Build history of the part. All positions in model axes, mm. A direction names the side the tool comes from. Give positions to 0.01 mm unless a question says otherwise; leave off trailing zeros. Write each loop counter-clockwise with the first axis right and the second up, starting at its lowest first coordinate (ties: lowest second). Pieces come first, ordered by that corner, then holes.
from build123d import *

# Parameters (mm, degrees)
SKETCH_1_R          = 20
SKETCH_1_R_2        = 5
SKETCH_1_R_3        = 2.25
EXTRUDE_1_DEPTH     = 6
SKETCH_2_R          = 9.5
SKETCH_2_R_2        = 5
EXTRUDE_2_DEPTH     = 23
SKETCH_3_R          = 3.75
CUT_EXTRUDE_1_DEPTH = 4.5


with BuildPart() as part:
    # Эскиз1 → Бобышка-Вытянуть1 (new body)
    with BuildSketch(Plane.XY):
        Circle(SKETCH_1_R)
        Circle(SKETCH_1_R_2, mode=Mode.SUBTRACT)
        with Locations((0, 14.5)):
            Circle(SKETCH_1_R_3, mode=Mode.SUBTRACT)
        with Locations((14.5, 0)):
            Circle(SKETCH_1_R_3, mode=Mode.SUBTRACT)
        with Locations((0, -14.5)):
            Circle(SKETCH_1_R_3, mode=Mode.SUBTRACT)
        with Locations((-14.5, 0)):
            Circle(SKETCH_1_R_3, mode=Mode.SUBTRACT)
    extrude(amount=EXTRUDE_1_DEPTH)

    # Эскиз2 → Бобышка-Вытянуть2 (add)
    with BuildSketch(Plane.XY.offset(6)):
        Circle(SKETCH_2_R)
        Circle(SKETCH_2_R_2, mode=Mode.SUBTRACT)
    extrude(amount=EXTRUDE_2_DEPTH)

    # Эскиз3 → Вырез-Вытянуть1 (cut)
    with BuildSketch(Plane(origin=(0, 0, 0), x_dir=(-1, 0, 0), z_dir=(0, 0, -1))):
        with Locations((0, 14.5)):
            Circle(SKETCH_3_R)
        with Locations((14.5, 0)):
            Circle(SKETCH_3_R)
        with Locations((0, -14.5)):
            Circle(SKETCH_3_R)
        with Locations((-14.5, 0)):
            Circle(SKETCH_3_R)
    extrude(amount=-CUT_EXTRUDE_1_DEPTH, mode=Mode.SUBTRACT)


solid = part.part
(1) Saw through at A-A, the plane x = 0. List the corners of the cut face in (y, z).
(2) Mould opens along X. For faces 4 (the face through (4, -9, 6)), 5 (the face through (13, -2, 4.5)), 6 (the face through (-4.336, -19.524, 2.958)) say: +X half, -X half, draft (parallel to the pull), parting line (faces both ways), or undercut.
(3) Probe line 1 (Y direction, x = 0, z = 2); line 2 (Y direction, x = 0, z = 4.9); line 3 (Z direction, x = -8.5, y = 12.5). List the from-to ranges inside material, lowest first.
(4) Drop flat-ended pins along their axis: pin 1 (8.5 mm diameter, centred on x = 14.5, y = 0, fed in from +Z); pin 2 (6 mm diameter, centred on x = -14.5, z = 6, fed in from -Y); pin 3 (5 mm diameter, centred on y = 11, z = 14, fed in from +X); pin 4 (3.5 mm diameter, centred on x = 0, y = -14.5, fed in from +Z). Give the stop position or say it passes through.
(5) Saw through at B-B, the plane y = 14.5. List the corners of the cut face in (x, z), plus the area to 3 significant figures.
(6) 3-axis set-ups, long thin cutter, end or side, ignore diameter. For faces 1 (the face through (-0.488, -16.696, 5.24)), 2 (the face through (4.38, -8.43, 17.34)), 3 (the face through (-2, -16, 4.5)): which of +Z, -Z, +X, -X, +Y, -Y reach the whole face in a straight line?
(7) Saw through at D-D, the plane z = 11.5. List the corners of the cut face in (x, y).
Computed values:
1. outline: (-20, 0) - (-18.25, 0) - (-18.25, 4.5) - (-16.75, 4.5) - (-16.75, 6) - (-20, 6) - close; (-12.25, 4.5) - (-10.75, 4.5) - (-10.75, 0) - (-5, 0) - (-5, 29) - (-9.5, 29) - (-9.5, 6) - (-12.25, 6) - close; (5, 0) - (10.75, 0) - (10.75, 4.5) - (12.25, 4.5) - (12.25, 6) - (9.5, 6) - (9.5, 29) - (5, 29) - close; (16.75, 4.5) - (18.25, 4.5) - (18.25, 0) - (20, 0) - (20, 6) - (16.75, 6) - close
2. face 4: draft
2. face 5: undercut
2. face 6: parting line
3. line 1: y = -20 to -18.25, -10.75 to -5, 5 to 10.75, 18.25 to 20
3. line 2: y = -20 to -16.75, -12.25 to -5, 5 to 12.25, 16.75 to 20
3. line 3: z = 0 to 6
4. pin 1: stops at z = 6
4. pin 2: stops at y = -16.36
4. pin 3: stops at x = 4.24
4. pin 4: passes through
5. outline: (-13.77, 0) - (-3.75, 0) - (-3.75, 4.5) - (-2.25, 4.5) - (-2.25, 6) - (-13.77, 6) - close; (2.25, 4.5) - (3.75, 4.5) - (3.75, 0) - (13.77, 0) - (13.77, 6) - (2.25, 6) - close
5. area: 125 mm2
6. face 1: +Z, -Z
6. face 2: +Z
6. face 3: -Z
7. outline: circle Ø19 at (0, 0); hole circle Ø10 at (0, 0)
